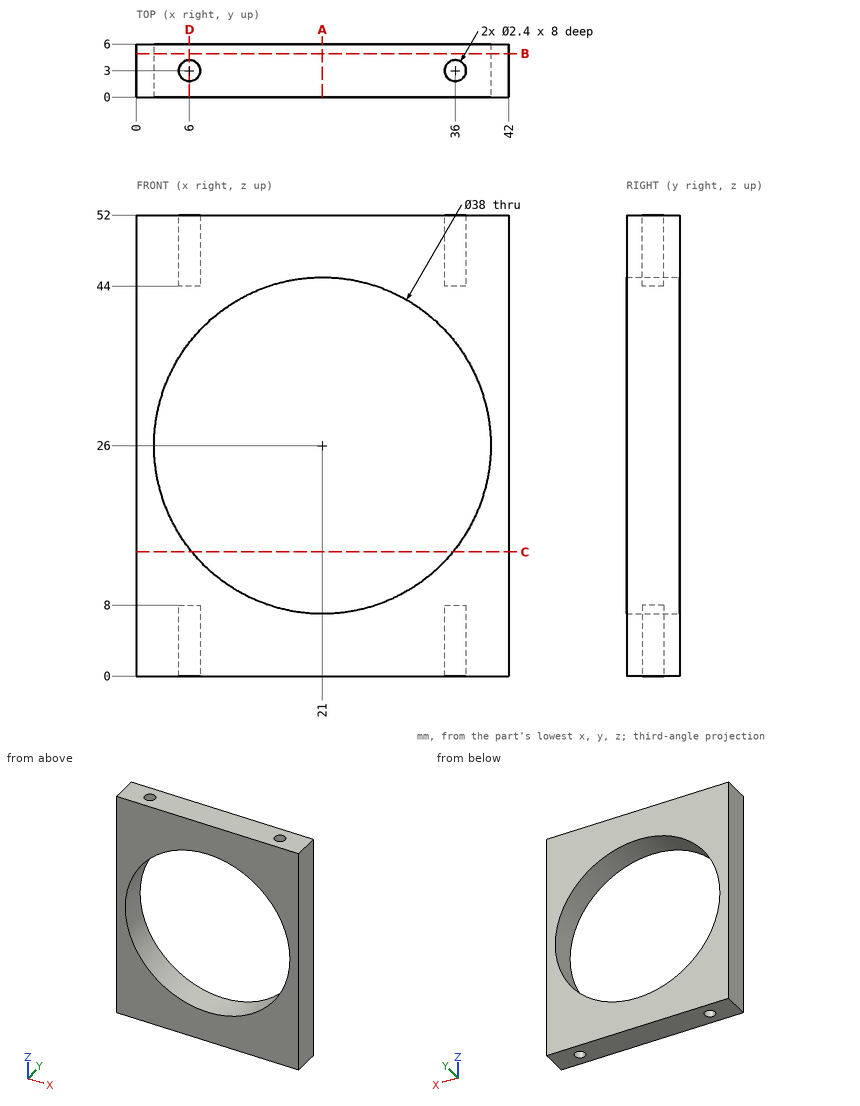
Input: dimensioned drawing with shaded views. Units: mm. Origin: part minimum x, y, z. Coordinates: 2 decimals unless noted, no trailing zeros. Loops run counter-clockwise (first coordinate to the right, second up) from the corner with the lowest first, then second, coordinate; pieces in that order, holes last. Notation, with made-up numbers: M 41.25,35 L 76.25,35 A31 cw 76.25,63 Z; hole C 20,-12 d7. An arc over 180 degrees is marked long. One line per item, written item: value. Start each with the question number.
1) Material intervals for L1, parallel to Y at x = 36, z = 2; L2, parallel to Z at x = 21, y = 3.05; L3, parallel to X at y = 0.65, z = 26.5, sorted ascending. Write a range as from..to.
2) Cut plane B-B (y = 4.9). Return loops of the section in (x, z), then the cut area to 3 significant figures.
3) Pin query (flat end, axial travel): P1, Ø0.7, axis at x = 36, y = 3, coming from the +Z side; P2, Ø8, axis at x = 17.5, z = 46, coming from the -Y side; P3, Ø2, axis at x = 6, y = 3, coming from the -Z side. Return the tip coordinate at first contact, or that it passes through.
4) Cut plane C-C (z = 14). Return loops of the section in (x, y).
5) Cut plane D-D (x = 6). Return loops of the section in (y, z).
6) Cut plane A-A (x = 21). Return loops of the section in (y, z).
Evaluation:
1. L1: 0..1.8, 4.2..6
1. L2: 0..7, 45..52
1. L3: 0..2.01, 39.99..42
2. outline: M 0,0 L 42,0 L 42,52 L 0,52 Z; hole C 21,26 d38
2. area: 1,050 mm^2
3. P1: z = 44
3. P2: y = 0
3. P3: z = 8
4. outline: M 0,0 L 6.27,0 L 6.27,6 L 0,6 Z; M 35.73,0 L 42,0 L 42,6 L 35.73,6 Z
5. outline: M 0,0 L 1.8,0 L 1.8,8 L 4.2,8 L 4.2,0 L 6,0 L 6,14.34 L 0,14.34 Z; M 0,37.66 L 6,37.66 L 6,52 L 4.2,52 L 4.2,44 L 1.8,44 L 1.8,52 L 0,52 Z
6. outline: M 0,0 L 6,0 L 6,7 L 0,7 Z; M 0,45 L 6,45 L 6,52 L 0,52 Z
